The model under review builds one solid part; all positions refer to its coordinate system, in mm. Face numbers are marked on the shaded views. A direction names the side the tool comes from. Give positions to 0.01 mm unless a question says otherwise; leave off trailing zeros. Loops run counter-clockwise (first coordinate to the right, second up) from the corner with the lowest first, then second, coordinate; pieces in that order, holes last. Notation, with made-up numbers: M 53,66 L 74,66 A23 cw 74,86 Z; hole C 17,0 d3. An arc over 180 degrees is marked long. Write item = value, one per line. Start each with the question number.
1. We need section B-B on z = 10.5. Give the boundary of the cut face in (x, y), then the cut area to 3 significant figures.
2. Wall thickness on line 1 along Y through (x, z) = (31, 20.25); line 2 along X through (y, z) = (17, 26); line 3 along Y through (x, z) = (49, 18): over which ranges is each line inside the solid? List them lowest first. Write a range as from..to.
3. We need section C-C on x = 29.5. Give the boundary of the cut face in (y, z).
4. For the marked faces 1, 2 and 3, list the 3-axis set-ups (+Z, -Z, +X, -X, +Y, -Y) from which the entire face can be reached by the end or side of a thin tool; tool diameter is ignored.
5. We need section A-A on z = 25. Give the boundary of the cut face in (x, y), then the cut area to 3 significant figures.
6. We need section D-D on z = 20.25. Give the boundary of the cut face in (x, y).
7. For pin 1 (4 mm diameter, centred on x = 19, y = 17.5, fed in from +Z); pin 2 (8 mm diameter, centred on y = 42, z = 6.5, fed in from +X); pin 3 (19 mm diameter, centred on x = 33.5, z = 24, fed in from +Y), all flat-tipped, find the tip position at first contact; note any pin that passes through.
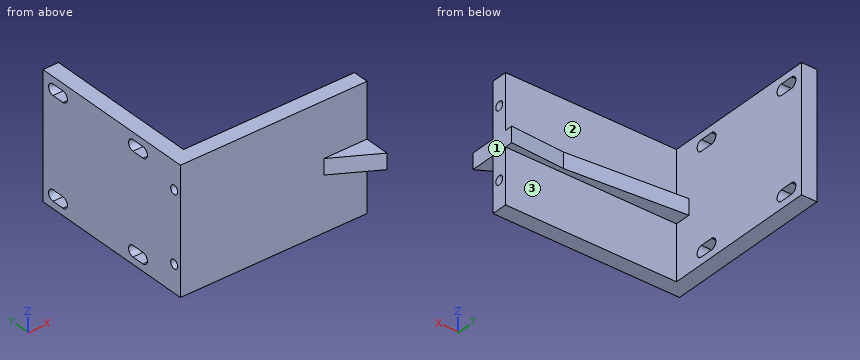
Autodesk Inventor part; units mm, degrees
ref_plane "YZ Plane" through (0, 0, 0) normal (1, 0, 0) x (0, 1, 0)
ref_plane "XZ Plane" through (0, 0, 0) normal (0, 1, 0) x (-1, 0, 0)
ref_plane "XY Plane" through (0, 0, 0) normal (0, 0, 1) x (1, 0, 0)
ref_plane "Arbeitsebene1" through (-0.5, 64.1414, -11) normal (-1, 0, 0) x (0, 0, 1)
sketch "Skizze1" plane through (-0.5, 64.1414, -11) normal (-1, 0, 0) x (0, 0, 1)
  line L0 (40, -27) -> (40, -40)
  line L1 (40, -27) -> (29, -27)
  line L2 (29, -40) -> (29, -27)
  line L3 (29, -40) -> (40, -40)
  circle A0 centre (32, -32) radius 1.5
  circle A1 centre (36, -36) radius 1.75
  line L4 (0, -40) -> (11, -40)
  line L5 (11, -40) -> (11, -27)
  line L6 (0, -27) -> (11, -27)
  line L7 (0, -27) -> (0, -40)
  circle A2 centre (8, -32) radius 1.5
  circle A3 centre (4, -36) radius 1.75
  line L8 (0, 0) -> (0, -13)
  line L9 (0, -13) -> (11, -13)
  line L10 (11, 0) -> (11, -13)
  line L11 (0, 0) -> (11, 0)
  circle A4 centre (8, -8) radius 1.5
  circle A5 centre (4, -4) radius 1.75
  line L12 (29, 0) -> (40, 0)
  line L13 (29, 0) -> (29, -13)
  line L14 (40, -13) -> (29, -13)
  line L15 (40, 0) -> (40, -13)
  circle A6 centre (32, -8) radius 1.5
  circle A7 centre (36, -4) radius 1.75
  line L16 (40, -40) -> (0, -40)
  line L17 (0, -40) -> (0, 0)
  line L18 (0, 0) -> (40, 0)
  line L19 (40, 0) -> (40, -40)
  line L20 (40, -40) -> (0, -40)
  line L21 (0, -40) -> (0, -55)
  line L22 (0, -55) -> (40, -55)
  line L23 (40, -55) -> (40, -40)
  line L24 (36, -36) -> (36, -40) construction
  line L25 (37.75, -36) -> (37.75, -40)
  line L26 (34.25, -40) -> (34.25, -36)
  arc A8 (37.75, -36) -> (34.25, -36) centre (36, -36) ccw
  arc A9 (34.25, -40) -> (37.75, -40) centre (36, -40) ccw
  line L27 (4, -36) -> (4, -40) construction
  line L28 (5.75, -36) -> (5.75, -40)
  line L29 (2.25, -40) -> (2.25, -36)
  arc A10 (5.75, -36) -> (2.25, -36) centre (4, -36) ccw
  arc A11 (2.25, -40) -> (5.75, -40) centre (4, -40) ccw
  line L30 (4, -4) -> (4, -8) construction
  line L31 (5.75, -4) -> (5.75, -8)
  line L32 (2.25, -8) -> (2.25, -4)
  arc A12 (5.75, -4) -> (2.25, -4) centre (4, -4) ccw
  arc A13 (2.25, -8) -> (5.75, -8) centre (4, -8) ccw
  line L33 (36, -4) -> (36, -8) construction
  line L34 (37.75, -4) -> (37.75, -8)
  line L35 (34.25, -8) -> (34.25, -4)
  arc A14 (37.75, -4) -> (34.25, -4) centre (36, -4) ccw
  arc A15 (34.25, -8) -> (37.75, -8) centre (36, -8) ccw
  point P0 (11, -64.1414)
  point P1 (40, -13)
  point P2 (0, -13)
  point P3 (0, -27)
  point P4 (0, -40)
  point P5 (36, -38)
  point P6 (4, -38)
  point P7 (4, -6)
  point P8 (36, -6)
  point P9 (37.75, -4)
  point P10 (34.25, -4)
  point P11 (5.75, -4)
  point P12 (2.25, -4)
  dimension "d0" = 15
extrude "Extrusion1" add sketch "Skizze1" along normal blind 5 contours L0 L3 L25 A1 L26 L2 L1 | L1 L2 L16 L5 L6 L17 L9 L10 L18 L13 L14 L19 | L23 L22 L21 L4 A11 L16 L3 A9 | L14 L13 L12 L15 | L4 L28 A3 L29 L7 L6 L5 | L10 L9 L8 L11 | A0 | A2 | A4 | A6
sketch "Skizze2" plane through (-0.5, 64.1414, -11) normal (1, 0, 0) x (0, 0, -1)
  line L0 (-40, -55) -> (-40, 0)
  line L1 (0, -55) -> (-40, -55)
  line L2 (0, 0) -> (0, -55)
  line L3 (-40, 0) -> (0, 0)
  arc A0 (-2.25, -36) -> (-5.75, -36) centre (-4, -36) ccw
  arc A1 (-2.25, -4) -> (-5.75, -4) centre (-4, -4) ccw
  arc A2 (-34.25, -4) -> (-37.75, -4) centre (-36, -4) ccw
  arc A3 (-34.25, -36) -> (-37.75, -36) centre (-36, -36) ccw
  line L4 (0, -55) -> (-40, -55)
  line L5 (-40, -55) -> (-40, -50)
  line L6 (-40, -50) -> (0, -50)
  line L7 (0, -50) -> (0, -55)
  line L8 (-2.25, -40) -> (-2.25, -36)
  arc A4 (-5.75, -40) -> (-2.25, -40) centre (-4, -40) ccw
  line L9 (-5.75, -36) -> (-5.75, -40)
  line L10 (-37.75, -4) -> (-37.75, -8)
  line L11 (-34.25, -8) -> (-34.25, -4)
  arc A5 (-37.75, -8) -> (-34.25, -8) centre (-36, -8) ccw
  line L12 (-34.25, -40) -> (-34.25, -36)
  arc A6 (-37.75, -40) -> (-34.25, -40) centre (-36, -40) ccw
  line L13 (-37.75, -36) -> (-37.75, -40)
  line L14 (-5.75, -4) -> (-5.75, -8)
  line L15 (-2.25, -8) -> (-2.25, -4)
  arc A7 (-5.75, -8) -> (-2.25, -8) centre (-4, -8) ccw
  point P0 (-11, -64.1414)
  dimension "d3" = 5
extrude "Extrusion2" add sketch "Skizze2" along normal blind 55 contours L0 L6 L2 L1
ref_plane "Arbeitsebene2" through (-0.5, 64.1414, 9) normal (0, 0, -1) x (-1, 0, 0)
sketch "Skizze3" plane through (-0.5, 64.1414, 9) normal (0, 0, -1) x (-1, 0, 0)
  line L0 (0, 0) -> (0, -50)
  line L1 (0, -50) -> (-55, -50)
  line L2 (-55, -55) -> (-55, -50)
  line L3 (5, -55) -> (-55, -55)
  line L4 (5, 0) -> (5, -55)
  line L5 (0, 0) -> (5, 0)
  line L6 (0, -50) -> (-55, -50)
  line L7 (-55, -50) -> (0, -45)
  line L8 (-55, -55) -> (-55, -50)
  line L9 (-55, -55) -> (-55, -63)
  line L10 (-55, -63) -> (-41.1436, -55)
  line L11 (-55, -55) -> (5, -55)
  line L12 (-41.1436, -55) -> (-55, -55)
  line L13 (-55, -50) -> (-55, -47.5)
  line L14 (-55, -47.5) -> (-37.6795, -48.4254)
  point P0 (-0.5, -64.1414)
  point P1 (-41.1436, -55)
  dimension "d7" = 5
  dimension "d14" = 8
  dimension "d15" = 60
extrude "Extrusion3" add sketch "Skizze3" along normal mid plane 5 contours L0 L1 L7 | L7 L13 L14 | L10 L9 L3
sketch "Skizze4" plane through (54.5, 64.1414, -11) normal (1, 0, 0) x (0, 0, -1)
  line L0 (-40, -50) -> (-40, -55)
  line L1 (-40, -55) -> (-22.5, -55)
  line L2 (0, -55) -> (0, -50)
  line L3 (-22.5, -50) -> (-40, -50)
  line L4 (0, -50) -> (-17.5, -50)
  circle A0 centre (-8.75, -52.5) radius 1.4
  circle A1 centre (-31.25, -52.5) radius 1.4
  line L5 (-22.5, -63) -> (-22.5, -55)
  line L6 (-17.5, -63) -> (-22.5, -63)
  line L7 (-17.5, -55) -> (-17.5, -63)
  line L8 (-17.5, -55) -> (0, -55)
  line L9 (-17.5, -47.5) -> (-17.5, -50)
  line L10 (-22.5, -47.5) -> (-17.5, -47.5)
  line L11 (-22.5, -50) -> (-22.5, -47.5)
  point P0 (-11, -64.1414)
  dimension "d10" = 2.8
  dimension "d11" = 2.8
extrude "Extrusion4" cut sketch "Skizze4" against normal through all contours A0 | A1
properties part number "40_XYZstage_micrometer_motorized_nema8_lightsheet_samplemount_ontop"
Final values:
q1.outline = M -5.5,9.14 L 40.64,9.14 L 54.5,1.14 L 54.5,16.64 L 37.18,15.72 L -0.5,19.14 L -0.5,64.14 L -5.5,64.14 Z
q1.area = 765 mm²
q2.line_1 = 9.14..10.24, 13.04..14.14
q2.line_2 = -5.5..-0.5
q2.line_3 = 9.14..14.14
q3.outline = M 9.14,-11 L 14.14,-11 L 14.14,6.5 L 16.41,6.5 L 16.41,11.5 L 14.14,11.5 L 14.14,29 L 9.14,29 Z; hole C 11.64,-2.25 d2.8; hole C 11.64,20.25 d2.8
q4.face_1 = +Z, -Z, +X, +Y, -Y
q4.face_2 = +Z, +X, +Y
q4.face_3 = -Z, +X, +Y
q5.outline = M -5.5,9.14 L 54.5,9.14 L 54.5,14.14 L -0.5,14.14 L -0.5,22.39 L -5.5,22.39 Z; M -5.5,29.89 L -0.5,29.89 L -0.5,54.39 L -5.5,54.39 Z; M -5.5,61.89 L -0.5,61.89 L -0.5,64.14 L -5.5,64.14 Z
q5.area = 475 mm²
q6.outline = M -5.5,9.14 L 54.5,9.14 L 54.5,10.24 L -5.5,10.24 Z; M -5.5,13.04 L 54.5,13.04 L 54.5,14.14 L -0.5,14.14 L -0.5,64.14 L -5.5,64.14 Z
q7.pin_1 = 11.5
q7.pin_2 = -0.5
q7.pin_3 = 14.14
